Read the model definition and answer for the solid it produces. Units are mm, in the model's axes. Coordinates: 2 decimals unless noted, no trailing zeros. Write each loop counter-clockwise with the first axis right and the second up, starting at its lowest first coordinate (ties: lowest second). Pieces come first, ordered by that corner, then holes.
1) The part is cut by section A-A (y = 40). Determine the outline of the cut face in (x, z).
2) The part is cut by section B-B (x = 0). Determine the outline of the cut face in (y, z).
3) The part is cut by section C-C (z = -0.3). Determine the outline of the cut face in (x, y), then the cut area to 3 significant figures.
4) Find the intervals of material crossed by line 1 (Y direction, x = 0, z = -0.25); line 2 (Y direction, x = -1.75, z = -0.9); line 3 (X direction, y = -0.5, z = -1), in increasing order.
from build123d import *

# Parameters (mm, degrees)
F0_W     = 10
F0_H     = 50
F0_R     = 2
F1_DEPTH = 2


with BuildPart() as f1:
    # F0 (on Top) → F1 (new body, symmetric)
    with BuildSketch(Plane.XY):
        with Locations((0, 20)):
            Rectangle(F0_W, F0_H)
        Circle(F0_R, mode=Mode.SUBTRACT)
        with Locations((0, 40)):
            Circle(F0_R, mode=Mode.SUBTRACT)
    extrude(amount=F1_DEPTH, both=True)


solid = f1.part
Reported:
1. outline: (-5, -2) - (-2, -2) - (-2, 2) - (-5, 2) - close; (2, -2) - (5, -2) - (5, 2) - (2, 2) - close
2. outline: (-5, -2) - (-2, -2) - (-2, 2) - (-5, 2) - close; (2, -2) - (38, -2) - (38, 2) - (2, 2) - close; (42, -2) - (45, -2) - (45, 2) - (42, 2) - close
3. outline: (-5, -5) - (5, -5) - (5, 45) - (-5, 45) - close; hole circle Ø4 at (0, 0); hole circle Ø4 at (0, 40)
3. area: 475 mm2
4. line 1: y = -5 to -2, 2 to 38, 42 to 45
4. line 2: y = -5 to -0.97, 0.97 to 39.03, 40.97 to 45
4. line 3: x = -5 to -1.94, 1.94 to 5
